Can you work these out from the model? Positions are in its coordinate system, mm. Coordinates: 2 decimals unless noted, no trailing zeros. Write each loop counter-clockwise with the first axis right and the second up, starting at its lowest first coordinate (ties: lowest second). Pieces come first, ordered by that corner, then holes.
```python
from build123d import *

# Parameters (mm, degrees)
SKETCH_1_W          = 147.5
SKETCH_1_H          = 68
EXTRUDE_1_DEPTH     = 2
SKETCH_2_W          = 2.1
SKETCH_2_H          = 15
EXTRUDE_2_DEPTH     = 2
SKETCH_3_R          = 1
CUT_EXTRUDE_1_DEPTH = 10
SKETCH_4_R          = 41
CUT_EXTRUDE_2_DEPTH = 86.383343966
SKETCH_5_W          = 7.55
SKETCH_5_H          = 56
CUT_EXTRUDE_3_DEPTH = 10
FILLET_1_R          = 1.5
SKETCH_6_R          = 1.6
CUT_EXTRUDE_4_DEPTH = 84.145790768


with BuildPart() as part:
    # 草图1 → 凸台-拉伸1 (new body)
    with BuildSketch(Plane.XY):
        Rectangle(SKETCH_1_W, SKETCH_1_H)
    extrude(amount=EXTRUDE_1_DEPTH)

    # 草图2 → 凸台-拉伸2 (add)
    with BuildSketch(Plane.XY.offset(2)):
        with Locations((-74.8, 0)):
            Rectangle(SKETCH_2_W, SKETCH_2_H)
    extrude(amount=-EXTRUDE_2_DEPTH)

    # 草图3 → 切除-拉伸1 (cut)
    with BuildSketch(Plane.XY.offset(2)):
        with Locations((-73.75, 8.5)):
            Circle(SKETCH_3_R)
        with Locations((-73.75, -8.5)):
            Circle(SKETCH_3_R)
    extrude(amount=-CUT_EXTRUDE_1_DEPTH, mode=Mode.SUBTRACT)

    # 草图4 → 切除-拉伸2 (cut, through all)
    with BuildSketch(Plane(origin=(0, -1.238963971, -15.184537967), x_dir=(-1, 0, 0), z_dir=(0, -0.08132352941176414, -0.9966877563028524))):
        with Locations((-26.25, -34.112616286)):
            Circle(SKETCH_4_R)
    extrude(amount=-CUT_EXTRUDE_2_DEPTH, mode=Mode.SUBTRACT)

    # 草图5 → 切除-拉伸3 (cut)
    with BuildSketch(Plane.XY.offset(2)):
        with BuildLine():
            ThreePointArc((57.2, 1.30806357), (61.228827839, -2.670411735), (64.75, -7.104491812))
            Line((64.75, -7.104491812), (64.75, 28))
            Line((64.75, 28), (57.2, 28))
            Line((57.2, 28), (57.2, 1.30806357))
        make_face()
        with BuildLine():
            ThreePointArc((43.65, 9.597715314), (47.51140105, 7.853227963), (51.2, 5.768068026))
            Line((51.2, 5.768068026), (51.2, 28))
            Line((51.2, 28), (43.65, 28))
            Line((43.65, 28), (43.65, 9.597715314))
        make_face()
        with BuildLine():
            ThreePointArc((30.1, 12.779255237), (33.900390726, 12.310383571), (37.65, 11.533697921))
            Line((37.65, 11.533697921), (37.65, 28))
            Line((37.65, 28), (30.1, 28))
            Line((30.1, 28), (30.1, 12.779255237))
        make_face()
        with BuildLine():
            ThreePointArc((16.55, 11.925357473), (20.3054817, 12.559762544), (24.1, 12.888005534))
            Line((24.1, 12.888005534), (24.1, 28))
            Line((24.1, 28), (16.55, 28))
            Line((16.55, 28), (16.55, 11.925357473))
        make_face()
        with BuildLine():
            Line((3, 28), (3, 6.783718345))
            ThreePointArc((3, 6.783718345), (6.698589297, 8.677613253), (10.55, 10.23743257))
            Line((10.55, 10.23743257), (10.55, 28))
            Line((10.55, 28), (3, 28))
        make_face()
        with BuildLine():
            Line((-10.55, 28), (-10.55, -4.826514156))
            ThreePointArc((-10.55, -4.826514156), (-6.990214832, -0.834971606), (-3, 2.726301758))
            Line((-3, 2.726301758), (-3, 28))
            Line((-3, 28), (-10.55, 28))
        make_face()
        with BuildLine():
            Line((-24.1, -28), (-20.357323082, -28))
            ThreePointArc((-20.357323082, -28), (-18.949835838, -21.179670039), (-16.55, -14.642185119))
            Line((-16.55, -14.642185119), (-16.55, 28))
            Line((-16.55, 28), (-24.1, 28))
            Line((-24.1, 28), (-24.1, -28))
        make_face()
        with Locations((-33.875, 0)):
            Rectangle(SKETCH_5_W, SKETCH_5_H)
        with Locations((-47.425, 0)):
            Rectangle(SKETCH_5_W, SKETCH_5_H)
        with Locations((-60.975, 0)):
            Rectangle(SKETCH_5_W, SKETCH_5_H)
    extrude(amount=-CUT_EXTRUDE_3_DEPTH, mode=Mode.SUBTRACT)

    # 圆角1
    fillet_1_edges = [part.edges().sort_by_distance(p)[0] for p in [
        (-14.749747441, -34, 0.999999977),
        (67.249747441, -34, 0.999999977),
        (-73.75, -34, 1),
        (-73.75, -9.5, 1),
        (-73.75, 9.5, 1),
        (-73.75, 34, 1),
        (73.75, 34, 1),
        (73.75, -34, 1),
        (57.2, 1.30806357, 1),
        (57.2, 28, 1),
        (64.75, 28, 1),
        (30.1, 12.779255237, 1),
        (30.1, 28, 1),
        (37.65, 28, 1),
        (37.65, 11.533697921, 1),
        (3, 6.783718345, 1),
        (3, 28, 1),
        (10.55, 28, 1),
        (10.55, 10.23743257, 1),
        (-20.357323082, -28, 1),
        (-24.1, -28, 1),
        (-24.1, 28, 1),
        (-16.55, 28, 1),
        (-16.55, -14.642185119, 1),
        (-51.2, -28, 1),
        (-51.2, 28, 1),
        (-43.65, 28, 1),
        (-43.65, -28, 1),
        (-64.75, 28, 1),
        (-57.2, 28, 1),
        (-57.2, -28, 1),
        (-64.75, -28, 1),
        (-37.65, -28, 1),
        (-37.65, 28, 1),
        (-30.1, 28, 1),
        (-30.1, -28, 1),
        (-10.55, -4.826514156, 1),
        (-10.55, 28, 1),
        (-3, 28, 1),
        (-3, 2.726301758, 1),
        (16.55, 11.925357473, 1),
        (16.55, 28, 1),
        (24.1, 28, 1),
        (24.1, 12.888005534, 1),
        (43.65, 9.597715314, 1),
        (43.65, 28, 1),
        (51.2, 28, 1),
        (51.2, 5.768068026, 1),
        (64.75, -7.104491812, 1),
    ]]
    fillet(fillet_1_edges, radius=FILLET_1_R)

    # 草图6 → 切除-拉伸4 (cut, through all)
    with BuildSketch(Plane.XY.offset(2)):
        with Locations((70.75, -2)):
            Circle(SKETCH_6_R)
        with Locations((70.75, 18)):
            Circle(SKETCH_6_R)
    extrude(amount=-CUT_EXTRUDE_4_DEPTH, mode=Mode.SUBTRACT)


solid = part.part
```
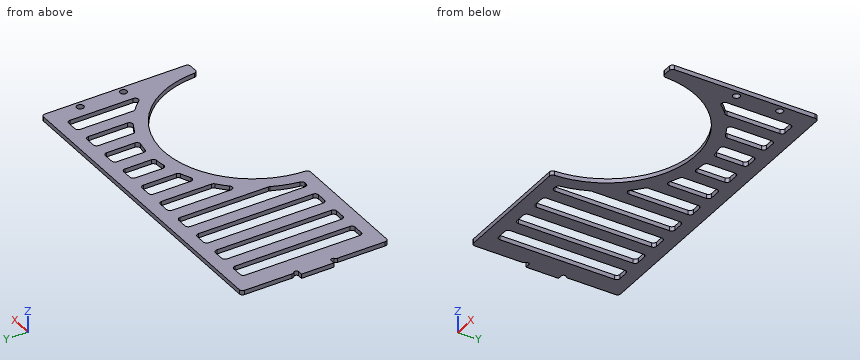
1. If we section it at C-C, the plane y = 18: Count the separate pieces of the cut face and the enclosed holes in it, plus the area to 3 significant figures.
2. If we section it at A-A, the plane x = 70.75: List the corners of the cut face in (y, z) for me.
3. If we section it at B-B, the plane x = 33.5: List the corners of the cut face in (y, z) for me.
4. If I drill on L1, parallel to Y at x = 70.75, z = 0.7; L2, parallel to Y at x = -63.5, z = 1.7; L3, parallel to X at y = -22, z = 0.3, over which ranges is the centre line in solid material (lowest first)?
5. I'm going to push flat-ended pins straight in: P1, Ø0.6, axis at y = 21.5, z = 1, coming from the -X side; P2, Ø1, axis at x = -46, y = -16.5, coming from the -Z side. Where does each tip first touch, or does it pass through?
Answers:
1. separate pieces: 12
1. enclosed holes: 0
1. area: 138 mm2
2. outline: (-34, 0) - (-3.6, 0) - (-3.6, 2) - (-34, 2) - close; (-0.4, 0) - (16.4, 0) - (16.4, 2) - (-0.4, 2) - close; (19.6, 0) - (34, 0) - (34, 2) - (19.6, 2) - close
3. outline: (6.26, 0) - (12.37, 0) - (12.37, 2) - (6.43, 2) - close; (28, 0) - (34, 0) - (34, 2) - (28, 2) - close
4. L1: y = -34 to -3.6, -0.4 to 16.4, 19.6 to 34
4. L2: y = -34 to -27.98, 27.98 to 34
4. L3: x = -73.75 to -64.75, -57.2 to -51.2, -43.65 to -37.65, -30.1 to -24.1, -19.18 to -12.9, 65.4 to 73.75
5. P1: stops at x = -73.75
5. P2: passes through
